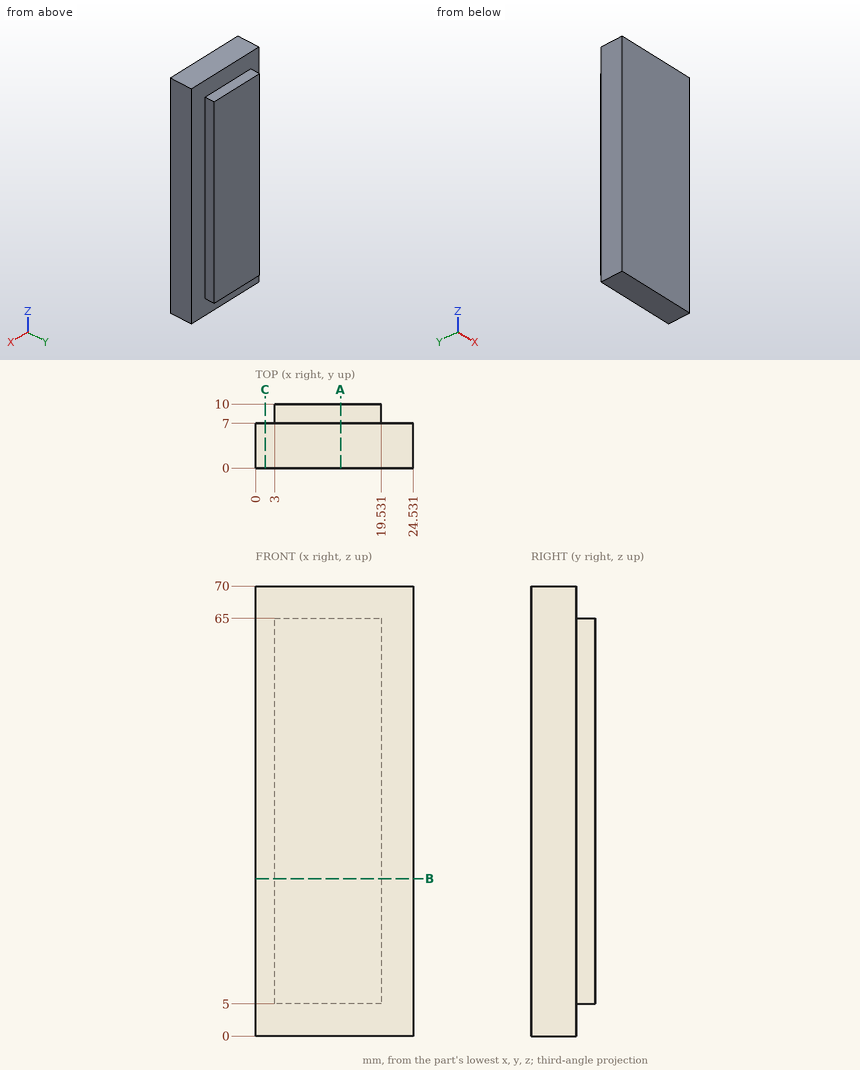
Source: three-view drawing plus pictorial views. Frame: mm from the lowest corner of the part. Round coordinates to 2 decimals unless told otherwise and drop trailing zeros. Order: outer loops, then holes, each group sorted by start corner. A loop starts at its lowest first (then second) coordinate and runs counter-clockwise, first axis right, second up. Notation, with made-up numbers: (61, 61.25) - (105, 61.25) arc R32 cw to (105, 93.25) - close; hole circle Ø7 at (62, 67). An arc over 180 degrees is marked (long way). Write each question's results on one line, items separated by ' | '.
Item 1: Section B-B, the plane z = 24.5. Return the cut outline in (x, y).
Completed:
outline: (0, 0) - (24.53, 0) - (24.53, 7) - (19.53, 7) - (19.53, 10) - (3, 10) - (3, 7) - (0, 7) - close
Item 2: Section C-C, the plane x = 1.5. Return the cut outline in (y, z).
Completed:
outline: (0, 0) - (7, 0) - (7, 70) - (0, 70) - close
Item 3: Section A-A, the plane x = 13.25. Return the cut outline in (y, z), and give its area (3 significant figures).
Completed:
outline: (0, 0) - (7, 0) - (7, 5) - (10, 5) - (10, 65) - (7, 65) - (7, 70) - (0, 70) - close | area: 670 mm^2
Item 4: Material intervals for line 1 along X through (y, z) = (9, 14.5); line 2 along Y through (x, z) = (1.5, 14); line 3 along Z through (x, y) = (13.5, 8.25), sorted ascending. Write a range as [from, to].
Completed:
line 1: [3, 19.53] | line 2: [0, 7] | line 3: [5, 65]
Item 5: First-contact query: pin 1 Ø3.5 at (x, y) = (10.5, 9) entering from -Z; pin 2 Ø2.5 at (y, z) = (9, 34) entering from +X. Flat tips, straight axial feed; report the tip coordinate or a pass-through.
Completed:
pin 1: z = 5 | pin 2: x = 19.53
